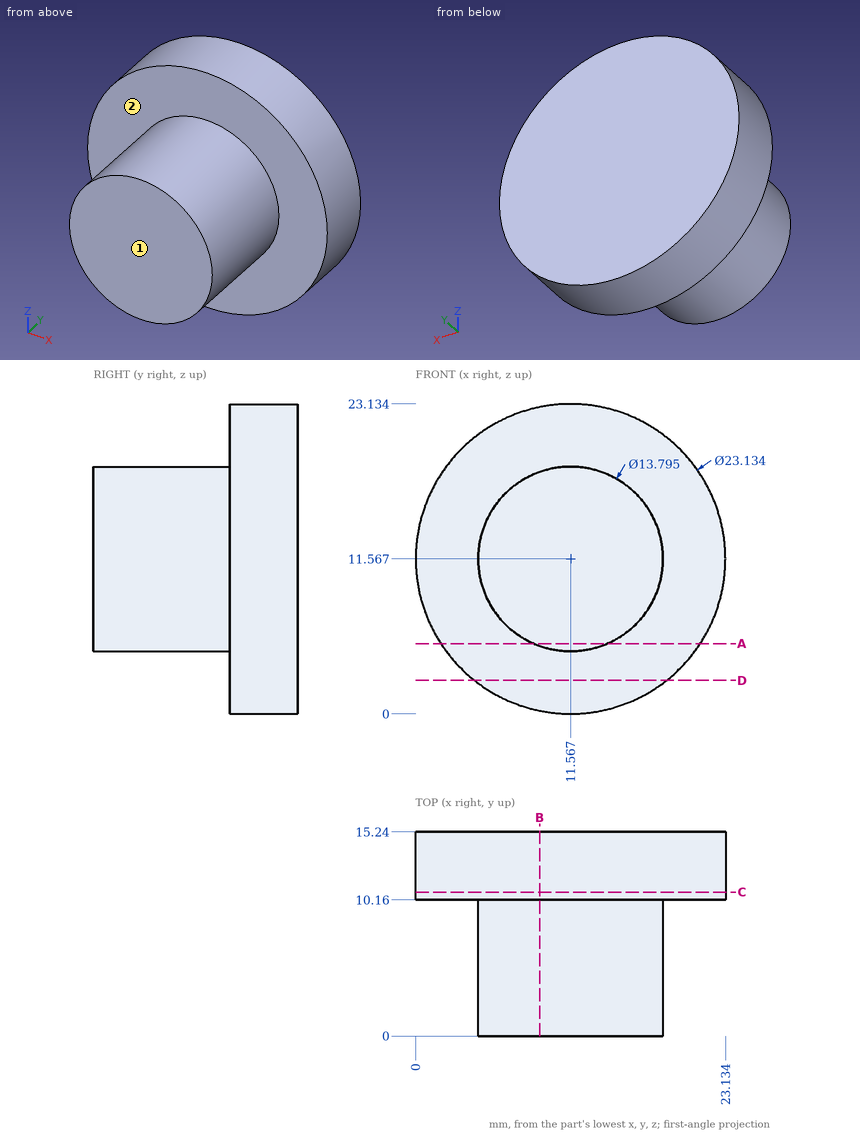
Print and shaded views of the part. All mm, measured from the part's lowest x, y and z. A direction names the side the tool comes from. Give positions to 0.01 mm unless a question says otherwise; leave off trailing zeros. Write each loop counter-clockwise with the first axis right and the second up, starting at its lowest first coordinate (ties: lowest second). Pieces come first, ordered by that corner, then holes. Notation, with made-up numbers: (-10, -6.75) -> (41, -6.75) arc R12 ccw to (41, 16.25) -> close; hole circle Ø10 at (-8.5, 34). An arc over 180 degrees is marked (long way). Write item = value, one per line.
(1) Probe line 1 along Y through (x, z) = (12.25, 4); line 2 along Z through (x, y) = (11.5, 11); line 3 along Z through (x, y) = (5.75, 12.25) (1 decimal). List the from-to ranges inside material, lowest first.
Determined:
line_1 = 10.16 to 15.24
line_2 = 0 to 23.13
line_3 = 1.6 to 21.6
(2) Tool access for the marked faces 1 and 2: list every direction of +Z, -Z, +X, -X, +Y, -Y with a clear straight run to the whole face (end or side of a thin tool).
Determined:
face_1 = +Z, -Z, +X, -X, -Y
face_2 = -Y
(3) Slice it at B-B, the plane x = 9.25. Give the cut face in (y, z) (1 decimal).
Determined:
outline = (0, 5.1) -> (10.2, 5.1) -> (10.2, 0.2) -> (15.2, 0.2) -> (15.2, 22.9) -> (10.2, 22.9) -> (10.2, 18.1) -> (0, 18.1) -> close
(4) Slice it at C-C, the plane y = 10.75. Give the cut face in (x, z), then the cut area to 3 significant figures.
Determined:
outline = circle Ø23.13 at (11.57, 11.57)
area = 420 mm2
(5) Slice it at D-D, the plane z = 2.5. Give the cut face in (x, y) (1 decimal).
Determined:
outline = (4.4, 10.2) -> (18.7, 10.2) -> (18.7, 15.2) -> (4.4, 15.2) -> close
(6) Flat gauge pins, fed straight in: P1, Ø5, axis at x = 15.5, y = 11, coming from the -Z side; P2, Ø1.5, axis at y = 4.5, z = 17, coming from the +X side; P3, Ø1, axis at y = 3, z = 17.5, coming from the -X side. Where does each tip first touch, or does it go through?
Determined:
P1 = 0.09
P2 = 16.63
P3 = 7.32
(7) Slice it at A-A, the plane z = 5.25. Give the cut face in (x, y), then the cut area to 3 significant figures.
Determined:
outline = (1.88, 10.16) -> (8.8, 10.16) -> (8.8, 0) -> (14.34, 0) -> (14.34, 10.16) -> (21.26, 10.16) -> (21.26, 15.24) -> (1.88, 15.24) -> close
area = 155 mm2
